Read the model definition and answer for the solid it produces. Units are mm, in the model's axes. A direction names the side the tool comes from. Round coordinates to 2 decimals unless told otherwise and drop trailing zeros. Loops run counter-clockwise (first coordinate to the right, second up) from the corner with the lowest first, then second, coordinate; pieces in that order, holes last. Notation, with made-up numbers: (88, 78) -> (109, 78) arc R22 ccw to (109, 86) -> close; hole circle Ø9 at (-3.75, 27.5). An arc over 180 degrees is marked (long way). Put each result on its own line as item: value.
from build123d import *


with BuildPart() as f1:
    # F0 (on Top) → F1 (revolve)
    with BuildSketch(Plane.XY):
        with BuildLine():
            Line((13.393199, 15.390105), (17.707892, 15.390105))
            Line((17.707892, 15.390105), (17.707892, 51.362158))
            Line((17.707892, 51.362158), (0, 51.362158))
            Line((0, 51.362158), (0, -1.483383))
            Line((0, -1.483383), (0, -28.184287))
            Line((0, -28.184287), (18.820429, -28.184287))
            Line((18.820429, -28.184287), (18.820429, -1.483383))
            Line((18.820429, -1.483383), (16.435054, -1.483383))
            ThreePointArc((16.435054, -1.483383), (17.135046, 7.353735), (13.393199, 15.390105))
        make_face()
    revolve(axis=Axis((0, 7.880475, 0), (0, -1, 0)))


solid = f1.part
Item 1: Which of the six approach directions +Z, -Z, +X, -X, +Y, -Y give full straight-line access (tool end or side, diameter ignored) to faces 3 (the cylindrical face through (-4.08, -14.647, -18.373)), 4 (the flat face through (13, 15.39, 4))?
Derived:
face 3: +Y, -Y
face 4: none
Item 2: The part is cut by section A-A (y = -9.5). Determine the outline of the cut face in (x, z), then the cut area to 3 significant figures.
Derived:
outline: circle Ø37.64 at (0, 0)
area: 1,110 mm^2
Item 3: For a pull along Z with two mould halves and no side action, classify faces 1 (the cylindrical face through (-13.05, 33.63, 11.97)), 2 (the flat face through (0, -28.184, 0)) as pulls with the +Z half, pulls with the -Z half, needs draft (parallel to the pull), parting line crosses it, or undercut.
Derived:
face 1: parting line crosses it
face 2: needs draft
Item 4: The part is cut by section B-B (z = 16.5). State how many separate pieces and enclosed holes the cut face has, then the cut area to 3 significant figures.
Derived:
separate pieces: 3
enclosed holes: 0
area: 1,040 mm^2
Item 5: Find the intervals of material crossed by line 1 along Z through (x, y) = (0, 20); line 2 along Y through (x, z) = (16, -7); line 3 along Y through (x, z) = (-3, -14), in increasing order.
Derived:
line 1: z = -17.71 to 17.71
line 2: y = -28.18 to -1.48, 15.39 to 51.36
line 3: y = -28.18 to 14.17, 15.39 to 51.36
Item 6: The part is cut by section C-C (y = 17). Determine the outline of the cut face in (x, z), then the cut area to 3 significant figures.
Derived:
outline: circle Ø35.42 at (0, 0)
area: 985 mm^2
Item 7: Flat-ended cylindrical pins translate along their axes: pin 1 Ø4 at (x, y) = (-5.5, -6.5) entering from -Z; pin 2 Ø10 at (x, y) = (10, -14.5) entering from +Z; pin 3 Ø5 at (x, y) = (4.5, -11.5) entering from -Z. Find the tip coordinate at first contact, or state that the pin passes through.
Derived:
pin 1: stops at z = -18.49
pin 2: stops at z = 18.14
pin 3: stops at z = -18.71
